Could you check a few things on this model? Use its own coordinates, in mm. Face numbers are marked on the shaded views. A direction names the side the tool comes from. Coordinates: 2 decimals unless noted, no trailing zeros. Write each loop counter-clockwise with the first axis right and the second up, starting at its lowest first coordinate (ties: lowest second). Pieces come first, ordered by that corner, then holes.
Item 1: For P1, Ø2, axis at y = 6, z = 24.5, coming from the +X side; P2, Ø4, axis at y = 11.5, z = 37, coming from the +X side; P3, Ø2, axis at y = 31, z = 15.5, coming from the +X side; P4, Ø4, axis at x = 35.5, y = 11.5, coming from the +Z side, each with a flat end and sliding along its axis, tell me the tip position at first contact or that it passes through.
Item 2: I want a section at B-B on y = 19.5. Please give me the cut outline in (x, z).
Item 3: I want a section at C-C on z = 9.5. Please give me the cut outline in (x, y).
Item 4: Which directions (+Z, -Z, +X, -X, +Y, -Y) give clear straight access to the entire face, cutting with the end or side of a thin tool? Please do the marked faces 1, 2 and 3.
Item 5: I want a section at D-D on x = 5. Please give me the cut outline in (y, z), then the cut area to 3 significant figures.
Item 6: If I drill on probe 1 along X at (y, z) = (16.5, 32); probe 2 along Z at (x, y) = (35, 12), over which ranges is the centre line in solid material (lowest first)?
Item 7: I want a section at A-A on x = 16. Please give me the cut outline in (y, z), then the cut area to 3 significant figures.
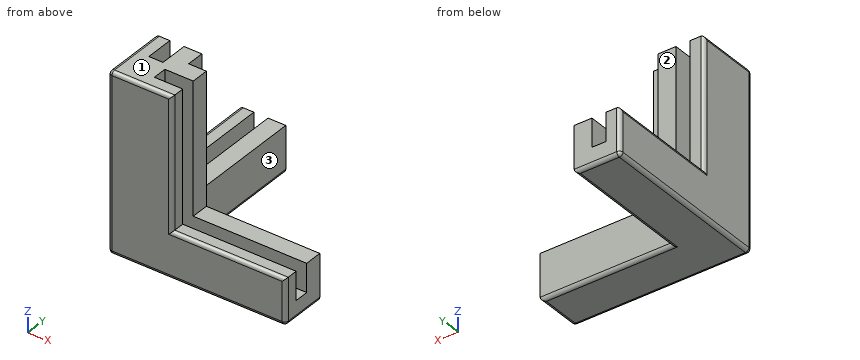
from build123d import *

# Parameters (mm, degrees)
PAD_DEPTH     = 13
PAD001_DEPTH  = 50
SKETCH002_W   = 70.608528
SKETCH002_H   = 4
SKETCH002_W_2 = 4
SKETCH002_H_2 = 60
POCKET_DEPTH  = 45
FILLET_R      = 1


with BuildPart() as part:
    # Sketch → Pad (new body)
    with BuildSketch(Plane.XY):
        Polygon((0, 0), (50, 0), (50, 13), (13, 13), (13, 50), (0, 50), align=None)
    extrude(amount=PAD_DEPTH)

    # Sketch001 → Pad001 (join)
    with BuildSketch(Plane.XY):
        Polygon((0, 0), (18, 0), (18, 13), (13, 13), (13, 18), (0, 18), align=None)
    extrude(amount=PAD001_DEPTH)

    # Sketch002 (on DatumPlane) → Pocket (cut)
    with BuildSketch(Plane.XY.offset(50)):
        with Locations((45.304264, 6)):
            Rectangle(SKETCH002_W, SKETCH002_H)
        with Locations((6, 40)):
            Rectangle(SKETCH002_W_2, SKETCH002_H_2)
    extrude(amount=-POCKET_DEPTH, mode=Mode.SUBTRACT)

    # Fillet
    fillet_edges = [part.edges().sort_by_distance(p)[0] for p in [
        (0, 25, 0),
        (6.5, 50, 0),
        (13, 31.5, 0),
        (31.5, 13, 0),
        (50, 6.5, 0),
        (25, 0, 0),
        (50, 0, 6.5),
        (34, 0, 13),
        (18, 0, 31.5),
        (9, 0, 50),
        (0, 0, 25),
        (0, 9, 50),
        (0, 18, 31.5),
        (0, 34, 13),
        (0, 50, 6.5),
    ]]
    fillet(fillet_edges, radius=FILLET_R)


solid = part.part
Response values:
1. P1: stops at x = 10
1. P2: stops at x = 18
1. P3: passes through
1. P4: stops at z = 13
2. outline: (0, 1) arc R1 ccw to (1, 0) - (12, 0) arc R1 ccw to (13, 1) - (13, 13) - (8, 13) - (8, 5) - (4, 5) - (4, 13) - (1, 13) arc R1 ccw to (0, 12) - close
3. outline: (0, 1) arc R1 ccw to (1, 0) - (49, 0) arc R1 ccw to (50, 1) - (50, 4) - (10, 4) - (10, 8) - (50, 8) - (50, 13) - (13, 13) - (13, 50) - (8, 50) - (8, 10) - (4, 10) - (4, 50) - (1, 50) arc R1 ccw to (0, 49) - close
4. face 1: +Z, +X, -X, +Y, -Y
4. face 2: +Z, +X, -X, +Y
4. face 3: +Z, -Z, +X, +Y
5. outline: (0, 1) arc R1 ccw to (1, 0) - (49, 0) arc R1 ccw to (50, 1) - (50, 5) - (10, 5) - (10, 50) - (1, 50) arc R1 ccw to (0, 49) - close
5. area: 699 mm2
6. probe 1: x = 0 to 4, 8 to 13
6. probe 2: z = 0 to 13
7. outline: (0, 1) arc R1 ccw to (1, 0) - (12, 0) arc R1 ccw to (13, 1) - (13, 50) - (8, 50) - (8, 5) - (4, 5) - (4, 50) - (1, 50) arc R1 ccw to (0, 49) - close
7. area: 469 mm2
